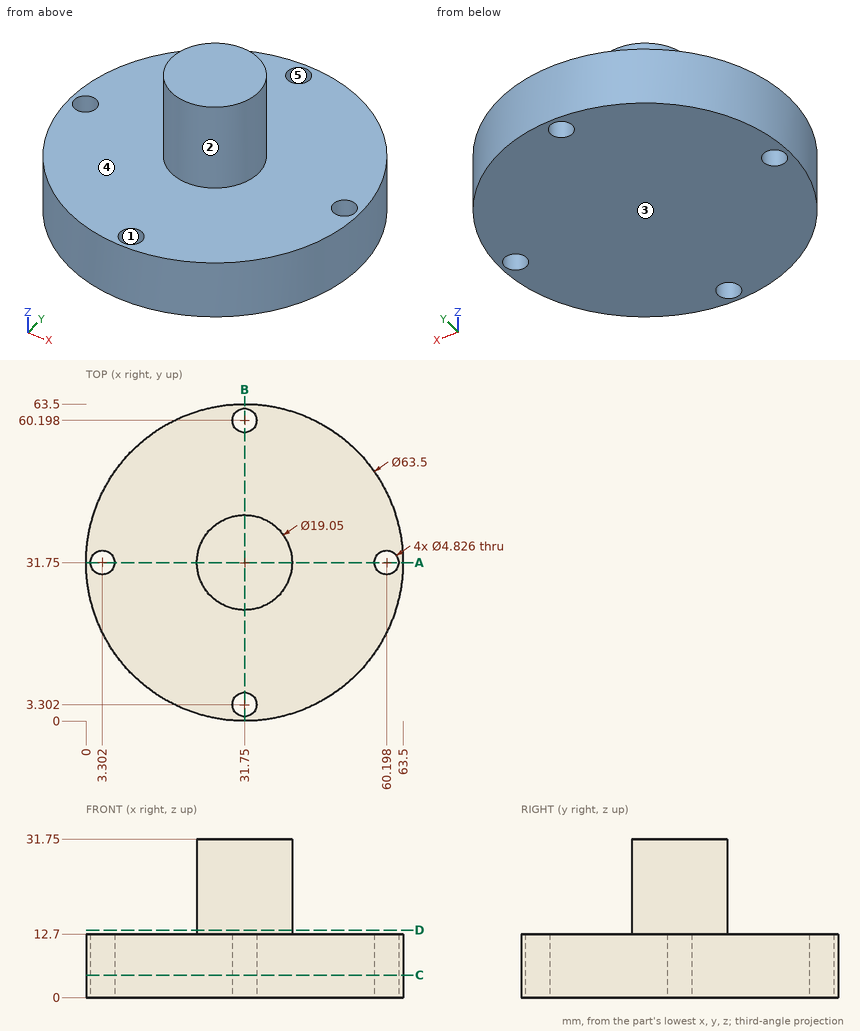
The drawing under review shows one solid part. Ordinate dimensions are in mm from its lowest x, y, z. A direction names the side the tool comes from. Coordinates: 2 decimals unless noted, no trailing zeros. Loops run counter-clockwise (first coordinate to the right, second up) from the corner with the lowest first, then second, coordinate; pieces in that order, holes last. Notation, with made-up numbers: (27.25, 81.5) -> (83.25, 81.5) arc R18 cw to (83.25, 102.5) -> close; hole circle Ø9 at (-23, -9). An arc over 180 degrees is marked (long way). Answer as a JSON object with one key per item and string values.
Q1. Tool access review of the marked faces 4 and 5: name each direction out of +Z, -Z, +X, -X, +Y, -Y from which nothing blocks a thin tool from reaching the whole face with its end or side.
Answer block:
{"face 4": "+Z", "face 5": "+Z, -Z"}
Q2. To check wall thickness, follow L1, parallel to X at y = 31, z = 7; L2, parallel to Z at x = 25, y = 52.5; L3, parallel to X at y = 5, z = 3.5. State the ranges of each line that lie inside material, in increasing order.
Answer block:
{"L1": "x = 0.01 to 1.01, 5.6 to 57.9, 62.49 to 63.49", "L2": "z = 0 to 12.7", "L3": "x = 14.65 to 30.04, 33.46 to 48.85"}
Q3. Take a section at A-A on y = 31.75. Give the boundary of the cut face in (x, z) (3 decimals).
Answer block:
{"outline": "(0, 0) -> (0.889, 0) -> (0.889, 12.7) -> (0, 12.7) -> close; (5.715, 0) -> (57.785, 0) -> (57.785, 12.7) -> (41.275, 12.7) -> (41.275, 31.75) -> (22.225, 31.75) -> (22.225, 12.7) -> (5.715, 12.7) -> close; (62.611, 0) -> (63.5, 0) -> (63.5, 12.7) -> (62.611, 12.7) -> close"}
Q4. Take a section at D-D on z = 13.5. Give the boundary of the cut face in (x, y) (3 decimals), plus the area to 3 significant figures.
Answer block:
{"outline": "circle Ø19.05 at (31.75, 31.75)", "area": "285 mm^2"}
Q5. Clearance check with flat-ended pins moving along their axes: pin 1 Ø10 at (x, z) = (8.5, 13.5) entering from +Y; pin 2 Ø12 at (x, y) = (28.5, 15.5) entering from +Z; pin 3 Ø6 at (x, z) = (17, 4.5) entering from +Y. State where each tip first meets the part, or that it passes through.
Answer block:
{"pin 1": "stops at y = 57.69", "pin 2": "stops at z = 12.7", "pin 3": "stops at y = 61.25"}
Q6. Take a section at C-C on z = 4.5. Give the boundary of the cut face in (x, y), plus the area to 3 significant figures.
Answer block:
{"outline": "circle Ø63.5 at (31.75, 31.75); hole circle Ø4.83 at (3.3, 31.75); hole circle Ø4.83 at (31.75, 3.3); hole circle Ø4.83 at (31.75, 60.2); hole circle Ø4.83 at (60.2, 31.75)", "area": "3,090 mm^2"}
Q7. The part is to be moulded in two halves that separate along Y. For the marked faces 1, 2 and 3, say which applies: +Y half, -Y half, draft (parallel to the pull), parting line (faces both ways), or undercut.
Answer block:
{"face 1": "undercut", "face 2": "parting line", "face 3": "draft"}
